from build123d import *

# Parameters (mm, degrees)
SKETCH1_R           = 6
BOSS_EXTRUDE1_DEPTH = 14
SKETCH2_R           = 2
CUT_EXTRUDE1_DEPTH  = 93.822411087
FILLET1_R           = 3


with BuildPart() as part:
    # Sketch1 → Boss-Extrude1 (new body)
    with BuildSketch(Plane.XY):
        with BuildLine():
            Line((0, -65), (-11, -65))
            Line((-11, -65), (-11, -72))
            Line((-11, -72), (-8, -75))
            Line((-8, -75), (9, -75))
            Line((9, -75), (9, 75))
            ThreePointArc((9, 75), (-4, 88), (-17, 75))
            Line((-17, 75), (0, -10))
            Line((0, -10), (0, -65))
        make_face()
        with Locations((-4, 75)):
            Circle(SKETCH1_R, mode=Mode.SUBTRACT)
    extrude(amount=BOSS_EXTRUDE1_DEPTH)

    # Sketch2 → Cut-Extrude1 (cut, through all)
    with BuildSketch(Plane(origin=(9, 0, 0), x_dir=(0, 0, -1), z_dir=(1, 0, 0))):
        with Locations((-7, 75)):
            Circle(SKETCH2_R)
    extrude(amount=-CUT_EXTRUDE1_DEPTH, mode=Mode.SUBTRACT)

    # Fillet1
    fillet1_edges = [part.edges().sort_by_distance(p)[0] for p in [
        (9, -75, 7),
    ]]
    fillet(fillet1_edges, radius=FILLET1_R)


solid = part.part
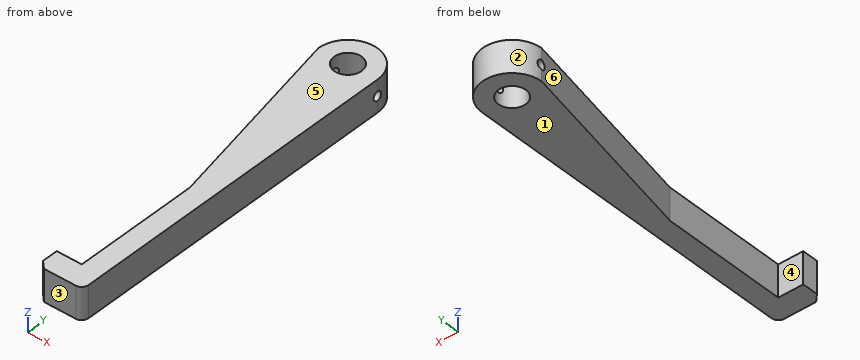
The listing builds one solid part. Answer for the finished solid, in the listing's coordinates (mm). Face numbers are marked on the shaded views. A direction names the side the tool comes from. Coordinates: 2 decimals unless noted, no trailing zeros. Write each loop counter-clockwise with the first axis right and the second up, starting at its lowest first coordinate (ties: lowest second). Pieces come first, ordered by that corner, then holes. Notation, with made-up numbers: (-15, 11.25) - (5, 11.25) arc R22 cw to (5, 26.25) - close; hole circle Ø11 at (65.25, -15). An arc over 180 degrees is marked (long way). Return JSON: item names as keys, results as strings.
1. Which of the six approach directions +Z, -Z, +X, -X, +Y, -Y give full straight-line access (tool end or side, diameter ignored) to the marked faces 5 and 6?
Final values:
{"face 5": "+Z, +X, -X, +Y, -Y", "face 6": "+Z, -Z, -X"}
2. Each of these flat-tipped pins is pushed along its axis until it touches: pin 1 Ø2 at (y, z) = (70, 7.5) entering from -X; pin 2 Ø1.5 at (x, z) = (-2, 11) entering from +Y; pin 3 Ø8 at (y, z) = (24, 10) entering from -X. Where does it stop, or does it pass through?
Final values:
{"pin 1": "x = -16.2", "pin 2": "y = 87.94", "pin 3": "x = -7.6"}
3. The part is cut by section D-D on x = -14. Determine the outline of the cut face in (y, z).
Final values:
{"outline": "(60, 0) - (83.31, 0) - (83.31, 14) - (60, 14) - close; hole circle Ø4 at (75, 7)"}
4. For a pull along Y with two mould halves and no side action, classify the marked faces 1, 2, 3 and 4 as +Y half, -Y half, draft (parallel to the pull), parting line (faces both ways), or undercut.
Final values:
{"face 1": "draft", "face 2": "+Y half", "face 3": "-Y half", "face 4": "undercut"}
5. The part is cut by section A-A on x = -4. Determine the outline of the cut face in (y, z), then the cut area to 3 significant figures.
Final values:
{"outline": "(-75, 0) - (-65, 0) - (-65, 14) - (-75, 14) - close; (10, 0) - (69, 0) - (69, 14) - (10, 14) - close; (81, 0) - (88, 0) - (88, 14) - (81, 14) - close", "area": "1,060 mm^2"}
6. The part is cut by section C-C on y = -46. Determine the outline of the cut face in (x, z).
Final values:
{"outline": "(0, 0) - (9, 0) - (9, 14) - (0, 14) - close"}
7. The part is cut by section B-B on z = 10.5. Determine the outline of the cut face in (x, y), then the cut area to 3 significant figures.
Final values:
{"outline": "(-17, 75) - (0, -10) - (0, -65) - (-11, -65) - (-11, -72) - (-8, -75) - (6, -75) arc R3 ccw to (9, -72) - (9, 75) arc R13 ccw to start; hole circle Ø12 at (-4, 75)", "area": "2,330 mm^2"}
8. Consider line 1 along X through (y, z) = (75, 4); line 2 along X through (y, z) = (-45.5, 7.25); line 3 along X through (y, z) = (51, 6). Determine where each line is inside the solid, lowest interval first.
Final values:
{"line 1": "-17 to -10, 2 to 9", "line 2": "0 to 9", "line 3": "-12.2 to 9"}
